Drawing for the job (mm, zero at the part's lowest x, y, z). A direction names the side the tool comes from. Give positions to 0.01 mm unless a question says otherwise; leave off trailing zeros. Write each loop counter-clockwise with the first axis right and the second up, starting at its lowest first coordinate (ties: lowest second). Pieces come first, ordered by that corner, then holes. Notation, with made-up numbers: (35.5, 62) - (84.5, 62) arc R21 cw to (84.5, 87) - close; hole circle Ø6 at (48.5, -3). An arc over 180 degrees is marked (long way). Use CSV: the item, a comma, the result in double quotes.
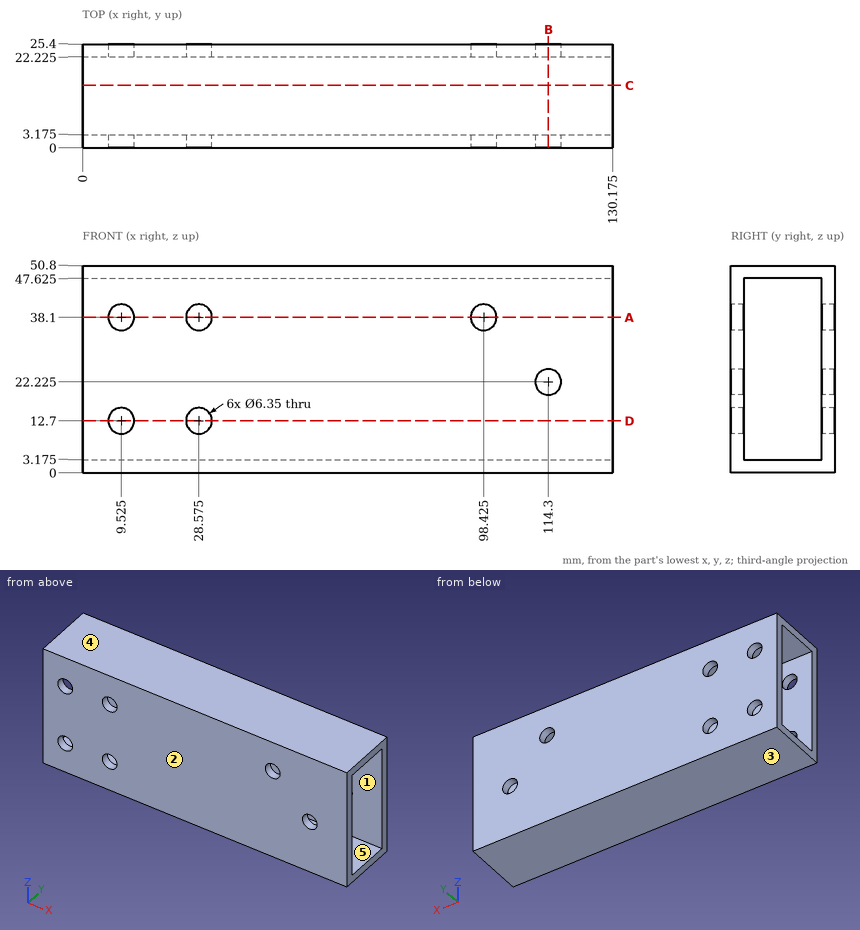
(1) Pull direction Y, two halves, no side cores. Call the marked faces 1, 2 and 3: released by +Y, released by -Y, zero draft, split by the parting line, or undercut.
Checked values:
face 1,"undercut"
face 2,"released by -Y"
face 3,"zero draft"
(2) 3-axis set-ups, long thin cutter, end or side, ignore diameter. For the marked faces 4 and 5: which of +Z, -Z, +X, -X, +Y, -Y reach the whole face in a straight line?
Checked values:
face 4,"+Z, +X, -X, +Y, -Y"
face 5,"+X, -X"
(3) Wall check: probe 1 along Y at (x, z) = (90, 19.5) (3 decimals); probe 2 along Z at (x, y) = (85, 9.75) (3 decimals); probe 3 along X at (y, z) = (23.25, 12) (3 decimals). Give the ranges that are in metal, low to high. Write a range as [from, to].
Checked values:
probe 1,"y = [0, 3.175], [22.225, 25.4]"
probe 2,"z = [0, 3.175], [47.625, 50.8]"
probe 3,"x = [0, 6.428], [12.622, 25.478], [31.672, 130.175]"
(4) Saw through at B-B, the plane x = 114.3. List the corners of the cut face in (y, z) (3 decimals).
Checked values:
outline,"(0, 0) - (25.4, 0) - (25.4, 19.05) - (22.225, 19.05) - (22.225, 3.175) - (3.175, 3.175) - (3.175, 19.05) - (0, 19.05) - close; (0, 25.4) - (3.175, 25.4) - (3.175, 47.625) - (22.225, 47.625) - (22.225, 25.4) - (25.4, 25.4) - (25.4, 50.8) - (0, 50.8) - close"
(5) Saw through at A-A, the plane z = 38.1. Count the separate pieces of the cut face and the enclosed holes in it, then the cut area to 3 significant figures.
Checked values:
separate pieces,"8"
enclosed holes,"0"
area,"706 mm^2"
(6) Saw through at C-C, the plane y = 15.25. List the corners of the cut face in (x, z) (3 decimals).
Checked values:
outline,"(0, 0) - (130.175, 0) - (130.175, 3.175) - (0, 3.175) - close; (0, 47.625) - (130.175, 47.625) - (130.175, 50.8) - (0, 50.8) - close"
(7) Saw through at D-D, the plane z = 12.7. List the corners of the cut face in (x, y) (3 decimals), then the cut area to 3 significant figures.
Checked values:
outline,"(0, 0) - (6.35, 0) - (6.35, 3.175) - (0, 3.175) - close; (0, 22.225) - (6.35, 22.225) - (6.35, 25.4) - (0, 25.4) - close; (12.7, 0) - (25.4, 0) - (25.4, 3.175) - (12.7, 3.175) - close; (12.7, 22.225) - (25.4, 22.225) - (25.4, 25.4) - (12.7, 25.4) - close; (31.75, 0) - (130.175, 0) - (130.175, 3.175) - (31.75, 3.175) - close; (31.75, 22.225) - (130.175, 22.225) - (130.175, 25.4) - (31.75, 25.4) - close"
area,"746 mm^2"
